The model under review builds one solid part; all positions refer to its coordinate system, in mm. A direction names the side the tool comes from. Coordinates: 2 decimals unless noted, no trailing zeros. Write each loop counter-clockwise with the first axis right and the second up, starting at its lowest first coordinate (ties: lowest second). Pieces come first, ordered by that corner, then holes. Notation, with made-up numbers: (74.25, 24) - (101.25, 24) arc R20 cw to (101.25, 52) - close; hole circle Ø7 at (-18, -26). An arc over 180 degrees is marked (long way). Put each result on its own line as item: value.
from build123d import *

# Parameters (mm, degrees)
BOSS_EXTRUDE1_DEPTH = 270
SHELL1_T            = -2


with BuildPart() as part:
    # Sketch1 → Boss-Extrude1 (new, symmetric)
    with BuildSketch(Plane(origin=(0, 0, 0), x_dir=(1, 0, 0), z_dir=(0, 1, 0))):
        with BuildLine():
            Line((-24, -30), (24, -30))
            ThreePointArc((24, -30), (28.242640687, -28.242640687), (30, -24))
            Line((30, -24), (30, 24))
            ThreePointArc((30, 24), (28.242640687, 28.242640687), (24, 30))
            Line((24, 30), (-24, 30))
            ThreePointArc((-24, 30), (-28.242640687, 28.242640687), (-30, 24))
            Line((-30, 24), (-30, -24))
            ThreePointArc((-30, -24), (-28.242640687, -28.242640687), (-24, -30))
        make_face()
    extrude(amount=BOSS_EXTRUDE1_DEPTH, both=True)

    # Shell1
    shell1_openings = [part.faces().sort_by_distance(p)[0] for p in [
        (0, 270, 0),
        (0, -270, 0),
    ]]
    offset(amount=SHELL1_T, openings=shell1_openings, kind=Kind.INTERSECTION)


solid = part.part
1. Machinability: for faces 5 (the flat face through (-30, 4, 0)), 6 (the flat face through (0, 4, -28)), which of the approach directions +Z, -Z, +X, -X, +Y, -Y give a long, thin tool a straight path to every point of the face, cutting with its end or side? Answer none if there is none.
Determined:
face 5: +Z, -Z, -X, +Y, -Y
face 6: +Y, -Y
2. Consider section C-C on y = 133.5. State the section outline as (x, z) points.
Determined:
outline: (-30, -24) arc R6 ccw to (-24, -30) - (24, -30) arc R6 ccw to (30, -24) - (30, 24) arc R6 ccw to (24, 30) - (-24, 30) arc R6 ccw to (-30, 24) - close; hole (-28, -24) arc R4 ccw to (-24, -28) - (24, -28) arc R4 ccw to (28, -24) - (28, 24) arc R4 ccw to (24, 28) - (-24, 28) arc R4 ccw to (-28, 24) - close
3. Consider section A-A on z = -8. State the section outline as (x, y) points.
Determined:
outline: (-30, -270) - (-28, -270) - (-28, 270) - (-30, 270) - close; (28, -270) - (30, -270) - (30, 270) - (28, 270) - close
4. For pin 1 Ø10 at (x, z) = (19, -11.5) entering from +Y, flat-tipped, find the tip position at first contact; note if it passes through.
Determined:
pin 1: passes through
5. The part is to be moulded in two halves that separate along Z. For faces 1 (the flat face through (0, 4, 30)), 2 (the flat face through (28, 4, 0)), 3 (the flat face through (0, 4, -30)), 4 (the flat face through (0, 4, 28)), say which applies: +Z half, -Z half, draft (parallel to the pull), parting line (faces both ways), or undercut.
Determined:
face 1: +Z half
face 2: undercut
face 3: -Z half
face 4: undercut
6. Consider section B-B on x = -19. State the section outline as (y, z) points, plus the area to 3 significant figures.
Determined:
outline: (-270, -30) - (270, -30) - (270, -28) - (-270, -28) - close; (-270, 28) - (270, 28) - (270, 30) - (-270, 30) - close
area: 2,160 mm^2
7. To check wall thickness, follow probe 1 along X at (y, z) = (-104, 19.5); probe 2 along Z at (x, y) = (27, -56.5). State the ranges of each line that lie inside material, in increasing order.
Determined:
probe 1: x = -30 to -28, 28 to 30
probe 2: z = -29.2 to -26.65, 26.65 to 29.2
